```python
from build123d import *

# Parameters (mm, degrees)
CHAMFER1_SIZE           = 0.75
SKETCH2_R               = 0.9
CUT_EXTRUDE1_DEPTH      = 4.3
CUT_EXTRUDE1_DEPTH_BACK = 4.3


with BuildPart() as part:
    # Sketch1 → Revolve1 (revolve)
    with BuildSketch(Plane.XY):
        Polygon((0, 16.5), (2.3, 16.5), (2.3, 1.5), (3.3, 1.5), (3.3, 0), (0, 0), align=None)
    revolve(axis=Axis((0, 0, 0), (0, 1, 0)))

    # Chamfer1
    chamfer1_edges = [part.edges().sort_by_distance(p)[0] for p in [
        (-2.3, 16.5, 0),
    ]]
    chamfer(chamfer1_edges, length=CHAMFER1_SIZE)

    # Sketch2 → Cut-Extrude1 (cut, two sides)
    with BuildSketch(Plane.XY) as cut_extrude1_sk:
        with Locations((0, 8.25)):
            Circle(SKETCH2_R)
    extrude(amount=CUT_EXTRUDE1_DEPTH, mode=Mode.SUBTRACT)
    extrude(cut_extrude1_sk.sketch, amount=-CUT_EXTRUDE1_DEPTH_BACK, mode=Mode.SUBTRACT)


solid = part.part
```
For this review, take the finished solid that the model builds, in its own axes (mm). A direction names the side the tool comes from. Give positions to 0.01 mm unless a question says otherwise; leave off trailing zeros. Order: outer loops, then holes, each group sorted by start corner. A loop starts at its lowest first (then second) coordinate and runs counter-clockwise, first axis right, second up.
1) Wall thickness on line 1 (Y direction, x = 0, z = -0.2); line 2 (X direction, y = 8.25, z = 0.1); line 3 (Y direction, x = 0.75, z = -2): over which ranges is each line inside the solid? List them lowest first.
2) For faces 1 (the face through (-2.43, 0.74, -2.23)), 2 (the face through (-1.4, 1.5, 2.2)), list the 3-axis set-ups (+Z, -Z, +X, -X, +Y, -Y) from which the entire face can be reached by the end or side of a thin tool; tool diameter is ignored.
3) Take a section at D-D (y = 12.5). Give the boundary of the cut face in (x, z).
4) Take a section at C-C (y = 8.25). Give the boundary of the cut face in (x, z).
5) Take a section at A-A (x = 0). Give the boundary of the cut face in (y, z), then the cut area to 3 significant figures.
6) Take a section at B-B (z = 0). Give the boundary of the cut face in (x, y), then the cut area to 3 significant figures.
7) The part is to be moulded in two halves that separate along Y. For faces 3 (the face through (0, 16.5, 0)), 4 (the face through (-0.12, 9.14, 0.03)), 5 (the face through (2.125, 8.525, 0.881)), say which applies: released by +Y, released by -Y, zero draft, split by the parting line, or undercut.
8) Insertion check: pin 1 (1 mm diameter, centred on y = 5.5, z = 1.5, fed in from -X); pin 2 (1 mm diameter, centred on y = 10, z = 2, fed in from -X); pin 3 (1.5 mm diameter, centred on x = 1.5, y = 12, fed in from -Z). Each pin has a flat end and moves straight along its axis. Give the tip position at first contact, or say it passes through.
Derived:
1. line 1: y = 0 to 7.35, 9.15 to 16.5
1. line 2: x = -2.3 to -0.9, 0.9 to 2.3
1. line 3: y = 0 to 7.75, 8.75 to 15.91
2. face 1: +Y, -Y
2. face 2: +Y
3. outline: circle Ø4.6 at (0, 0)
4. outline: (-0.9, -2.12) - (-0.9, 2.12) arc R2.3 ccw to start; (0.9, -2.12) arc R2.3 ccw to (0.9, 2.12) - close
5. outline: (0, -3.3) - (1.5, -3.3) - (1.5, -2.3) - (7.35, -2.3) - (7.35, 2.3) - (1.5, 2.3) - (1.5, 3.3) - (0, 3.3) - close; (9.15, -2.3) - (15.75, -2.3) - (16.5, -1.55) - (16.5, 1.55) - (15.75, 2.3) - (9.15, 2.3) - close
5. area: 70.1 mm2
6. outline: (-3.3, 0) - (3.3, 0) - (3.3, 1.5) - (2.3, 1.5) - (2.3, 15.75) - (1.55, 16.5) - (-1.55, 16.5) - (-2.3, 15.75) - (-2.3, 1.5) - (-3.3, 1.5) - close; hole circle Ø1.8 at (0, 8.25)
6. area: 75.8 mm2
7. face 3: released by +Y
7. face 4: undercut
7. face 5: zero draft
8. pin 1: stops at x = -2.07
8. pin 2: stops at x = -1.74
8. pin 3: stops at z = -2.17
